Source: three-view drawing plus pictorial views. Frame: mm from the lowest corner of the part. A direction names the side the tool comes from. Give positions to 0.01 mm unless a question says otherwise; leave off trailing zeros. Write each loop counter-clockwise with the first axis right and the second up, starting at its lowest first coordinate (ties: lowest second). Pieces come first, ordered by that corner, then holes.
Q1. Cut plane D-D on x = 5.25. Return the cut outline in (y, z).
Q2. Cut plane A-A on z = 2. Return the cut outline in (x, y).
Q3. Reachability of the marked faces 1, 2, 3 and 4 from +Z, -Z, +X, -X, +Y, -Y: full face, straight path, thin tool, end or side. Return the list, or none.
Q4. Line query: L1, parallel to Y at x = 15.5, z = 7.5; L2, parallel to Z at x = 5.25, y = 28.75; L3, parallel to Y at x = 13.5, z = 4. Output: solid intervals per line, ascending.
Q5. Cut plane C-C on z = 30.85. Return the cut outline in (x, y).
Q6. Pin query (flat end, axial travel): pin 1 (8.5 mm diameter, centred on x = 5.5, z = 28.5, fed in from +Y); pin 2 (5.5 mm diameter, centred on x = 5.25, z = 30.85, fed in from -Y); pin 3 (8 mm diameter, centred on x = 8, y = 42.5, fed in from -Z). Return the tip coordinate at first contact, or that it passes through.
Q7. Cut plane B-B on x = 10.5. Return the cut outline in (y, z), plus the area to 3 significant figures.
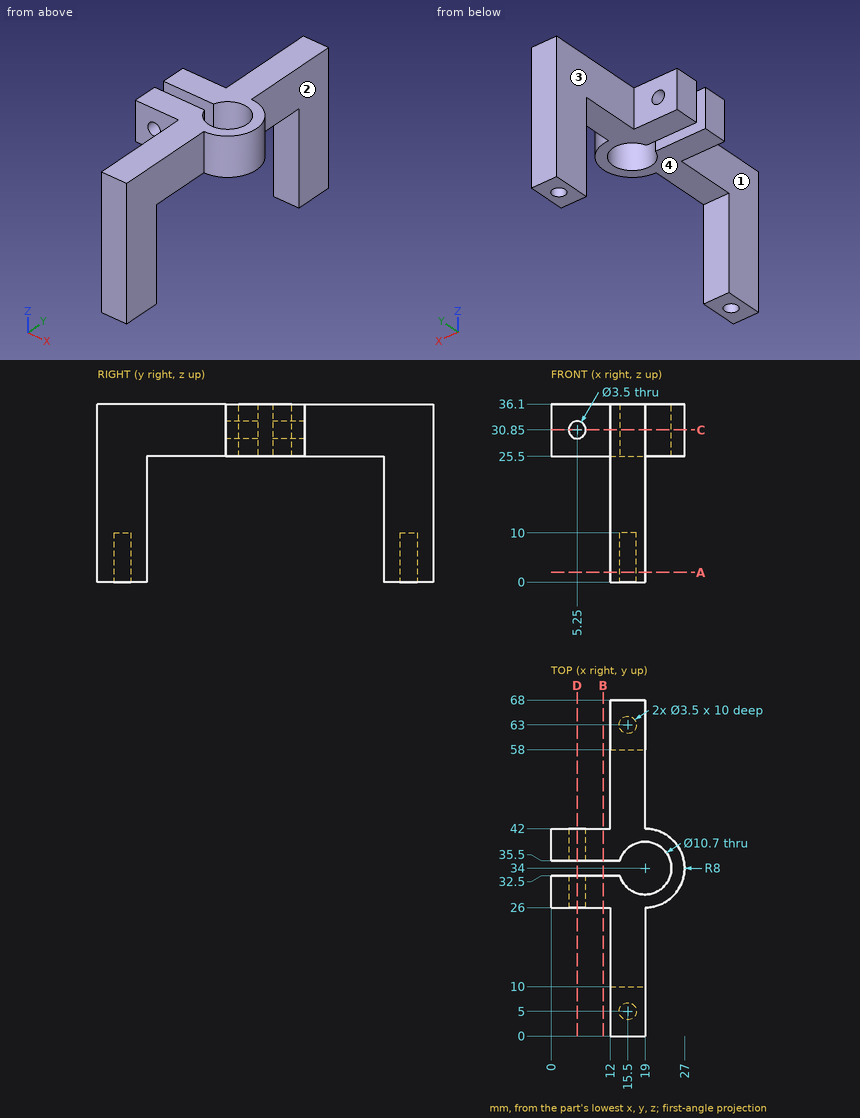
Data:
1. outline: (26, 25.5) - (32.5, 25.5) - (32.5, 29.1) - (26, 29.1) - close; (26, 32.6) - (32.5, 32.6) - (32.5, 36.1) - (26, 36.1) - close; (35.5, 25.5) - (42, 25.5) - (42, 29.1) - (35.5, 29.1) - close; (35.5, 32.6) - (42, 32.6) - (42, 36.1) - (35.5, 36.1) - close
2. outline: (12, 0) - (19, 0) - (19, 10) - (12, 10) - close; (12, 58) - (19, 58) - (19, 68) - (12, 68) - close; hole circle Ø3.5 at (15.5, 5); hole circle Ø3.5 at (15.5, 63)
3. face 1: +Z, -Z, -X, -Y
3. face 2: +Z, -Z, +X, +Y
3. face 3: +Z, -Z, -X, +Y
3. face 4: -Z, +X, -X
4. L1: y = 0 to 3.25, 6.75 to 10, 58 to 61.25, 64.75 to 68
4. L2: z = 25.5 to 29.1, 32.6 to 36.1
4. L3: y = 0 to 10, 58 to 68
5. outline: (0, 26) - (3.5, 26) - (3.5, 32.5) - (0, 32.5) - close; (0, 35.5) - (3.5, 35.5) - (3.5, 42) - (0, 42) - close; (7, 26) - (12, 26) - (12, 0) - (19, 0) - (19, 26) arc R8 ccw to (19, 42) - (19, 68) - (12, 68) - (12, 42) - (7, 42) - (7, 35.5) - (13.86, 35.5) arc R5.35 cw (long way) to (13.86, 32.5) - (7, 32.5) - close
6. pin 1: stops at y = 42
6. pin 2: stops at y = 26
6. pin 3: stops at z = 25.5
7. outline: (26, 25.5) - (32.5, 25.5) - (32.5, 36.1) - (26, 36.1) - close; (35.5, 25.5) - (42, 25.5) - (42, 36.1) - (35.5, 36.1) - close
7. area: 138 mm2
